The drawing under review shows one solid part. Ordinate dimensions are in mm from its lowest x, y, z. A direction names the side the tool comes from. Coordinates: 2 decimals unless noted, no trailing zeros. Order: outer loops, then holes, each group sorted by start corner. A loop starts at its lowest first (then second) coordinate and runs counter-clockwise, first axis right, second up.
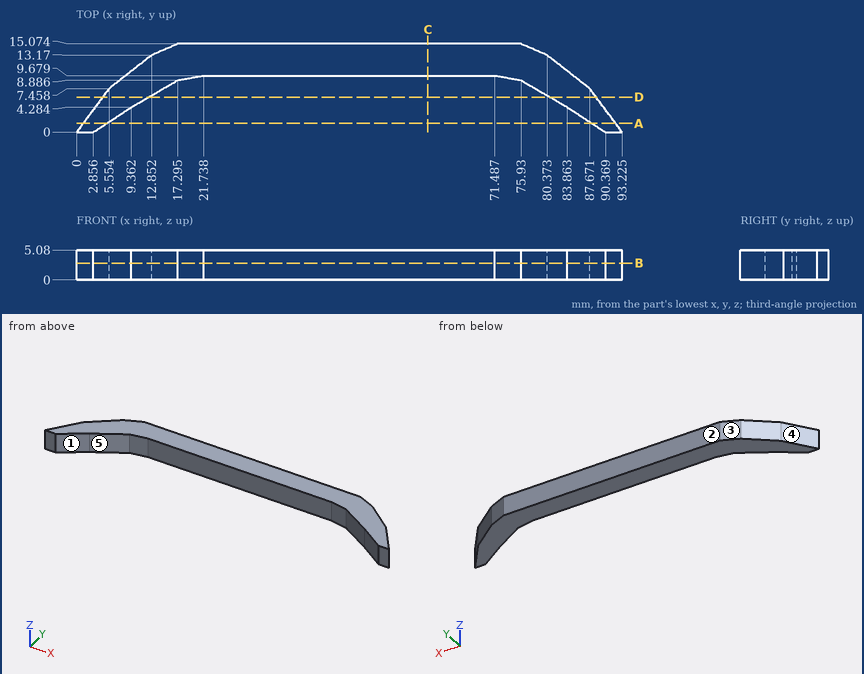
1. Add section C-C (x = 60). Give the boundary of the cut face in (y, z).
2. Add section D-D (y = 6). Give the boundary of the cut face in (x, z) (1 decimal).
3. To check wall thickness, follow line 1 (Y direction, x = 71.5, z = 4.8) (1 decimal); line 2 (X direction, y = 6, z = 0.4) (1 decimal); line 3 (X direction, y = 8.5, z = 1.6) (1 decimal). State the ranges of each line that lie inside material, in increasing order.
4. Mouldability with a two-part tool opening along X and no side actions: class the marked faces 1, 2 and 3 as pulls with the +X half, pulls with the -X half, needs draft (parallel to the pull), parting line crosses it, or undercut.
5. For the marked faces 4 and 5, list the 3-axis set-ups (+Z, -Z, +X, -X, +Y, -Y) from which the entire face can be reached by the end or side of a thin tool; tool diameter is ignored.
6. Insertion check: pin 1 (1.5 mm diameter, centred on x = 56.5, z = 2.5, fed in from -Y); pin 2 (1 mm diameter, centred on y = 5, z = 4.5, fed in from +X) (1 decimal). Each pin has a flat end and moves straight along its axis. Give the tip position at first contact, or say it passes through.
7. Add section A-A (y = 1.5). Give the boundary of the cut face in (x, z).
8. Add section B-B (z = 2.9). Give the boundary of the cut face in (x, y) (1 decimal).
Solution:
1. outline: (9.68, 0) - (15.07, 0) - (15.07, 5.08) - (9.68, 5.08) - close
2. outline: (4.5, 0) - (12.3, 0) - (12.3, 5.1) - (4.5, 5.1) - close; (80.9, 0) - (88.8, 0) - (88.8, 5.1) - (80.9, 5.1) - close
3. line 1: y = 9.7 to 15.1
3. line 2: x = 4.5 to 12.3, 80.9 to 88.8
3. line 3: x = 6.9 to 16.6, 76.6 to 86.3
4. face 1: undercut
4. face 2: needs draft
4. face 3: pulls with the -X half
5. face 4: +Z, -Z, -X, +Y
5. face 5: +Z, -Z, -Y
6. pin 1: stops at y = 9.68
6. pin 2: stops at x = 89.9
7. outline: (1.12, 0) - (5.13, 0) - (5.13, 5.08) - (1.12, 5.08) - close; (88.09, 0) - (92.11, 0) - (92.11, 5.08) - (88.09, 5.08) - close
8. outline: (0, 0) - (2.9, 0) - (9.4, 4.3) - (17.3, 8.9) - (21.7, 9.7) - (71.5, 9.7) - (75.9, 8.9) - (83.9, 4.3) - (90.4, 0) - (93.2, 0) - (87.7, 7.5) - (80.4, 13.2) - (75.9, 15.1) - (17.3, 15.1) - (12.9, 13.2) - (5.6, 7.5) - close
